Build history of the part. All positions in model axes, mm. Round coordinates to 2 decimals unless told otherwise and drop trailing zeros. Write each loop counter-clockwise with the first axis right and the second up, starting at its lowest first coordinate (ties: lowest second). Pieces come first, ordered by that corner, then holes. Notation, with made-up numbers: M 59,5.25 L 100,5.25 A30 ccw 100,33.25 Z; hole C -9,40 d6. An arc over 180 degrees is marked long. Use a Markdown table: item, result.
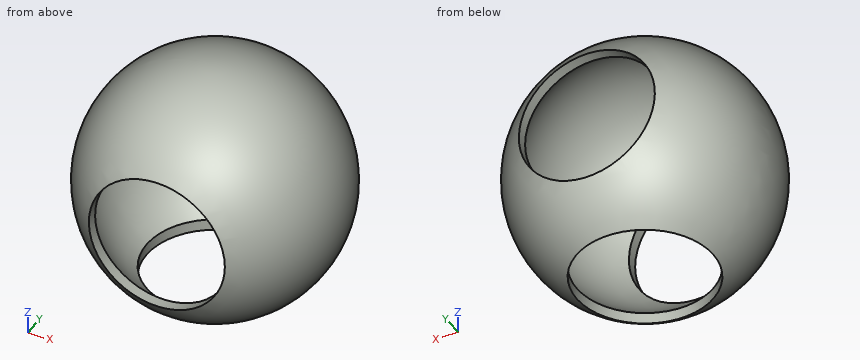
from build123d import *

# Parameters (mm, degrees)
F2_R          = 21.5
F3_DEPTH      = 40.001
F3_DEPTH_BACK = 40.001
F4_R          = 21.5
F5_DEPTH      = 40.001


with BuildPart() as f1:
    # F0 (on Front) → F1 (revolve)
    with BuildSketch(Plane.XZ):
        with BuildLine():
            Line((0, 37), (0, 40))
            ThreePointArc((0, 40), (-40, 0), (0, -40))
            Line((0, -40), (0, -37))
            ThreePointArc((0, -37), (-37, 0), (0, 37))
        make_face()
    revolve(axis=Axis((0, 0, -38.5), (0, 0, -1)))

    # F2 (on Front) → F3 (cut, two sides)
    with BuildSketch(Plane.XZ) as f3_sk:
        Circle(F2_R)
    extrude(amount=F3_DEPTH, mode=Mode.SUBTRACT)
    extrude(f3_sk.sketch, amount=-F3_DEPTH_BACK, mode=Mode.SUBTRACT)

    # F4 (on Top) → F5 (cut, through all)
    with BuildSketch(Plane.XY):
        Circle(F4_R)
    extrude(amount=-F5_DEPTH, mode=Mode.SUBTRACT)


solid = f1.part
Q1. Cut at A-A on x = 0. Give the cut face in (y, z).
Response values:
| item | result |
|---|---|
| outline | M -33.73,-21.5 A40 ccw -21.5,-33.73 L -21.5,-30.11 A37 cw -30.11,-21.5 Z; M -33.73,21.5 L -30.11,21.5 A37 cw 30.11,21.5 L 33.73,21.5 A40 ccw Z; M 21.5,-33.73 A40 ccw 33.73,-21.5 L 30.11,-21.5 A37 cw 21.5,-30.11 Z |
Q2. Drop flat-ended pins along their axis: P1, Ø1, axis at x = 13, y = -9.5, coming from the -Z side; P2, Ø3, axis at y = -26.5, z = 15, coming from the -X side; P3, Ø4, axis at x = -3, z = -25, coming from the +Y side; P4, Ø1.5, axis at x = 19, z = -7, coming from the -Y side. Give the stop position or say it passes through.
Response values:
| item | result |
|---|---|
| P1 | stops at z = 33.07 |
| P2 | stops at x = -27.6 |
| P3 | stops at y = 32.6 |
| P4 | passes through |
Q3. Drill centre lines: L1, parallel to X at y = -31, z = -3.5; L2, parallel to X at y = -31, z = 0; L3, parallel to Y at x = 27, z = 13.5. Where is each one in solid material? Low to high.
Response values:
| item | result |
|---|---|
| L1 | x = -25.03 to -21.21, 21.21 to 25.03 |
| L2 | x = -25.28 to -21.5, 21.5 to 25.28 |
| L3 | y = -26.24 to -21.4, 21.4 to 26.24 |
Q4. Cut at B-B on z = 0. Give the cut face in (x, y), and give its area (3 significant figures).
Response values:
| item | result |
|---|---|
| outline | M -21.5,-33.73 L -21.5,-30.11 A37 cw -21.5,30.11 L -21.5,33.73 A40 ccw Z; M 21.5,-33.73 A40 ccw 21.5,33.73 L 21.5,30.11 A37 cw 21.5,-30.11 Z |
| area | 452 mm2 |
Q5. Cut at D-D on y = 0. Give the cut face in (x, z).
Response values:
| item | result |
|---|---|
| outline | M -21.5,-33.73 L -21.5,-30.11 A37 cw long 21.5,-30.11 L 21.5,-33.73 A40 ccw long Z |
Q6. Cut at C-C on x = -17. Give the cut face in (y, z).
Response values:
| item | result |
|---|---|
| outline | M -33.73,-13.16 A36.21 ccw -13.16,-33.73 L -13.16,-30.11 A32.86 cw -30.11,-13.16 Z; M -33.73,13.16 L -30.11,13.16 A32.86 cw 30.11,13.16 L 33.73,13.16 A36.21 ccw Z; M 13.16,-33.73 A36.21 ccw 33.73,-13.16 L 30.11,-13.16 A32.86 cw 13.16,-30.11 Z |
